Design review of the part built by this model. Coordinates are the model's own, in mm. Face numbers are marked on the shaded views. A direction names the side the tool comes from. Coordinates: 2 decimals unless noted, no trailing zeros. Order: outer loops, then holes, each group sorted by start corner. A loop starts at its lowest first (then second) coordinate and runs counter-clockwise, first axis right, second up. Notation, with made-up numbers: (30, -7) -> (65, -7) arc R21 cw to (65, 25) -> close; hole circle Ø2 at (71, -13). An arc over 180 degrees is marked (long way). Write item = value, one per line.
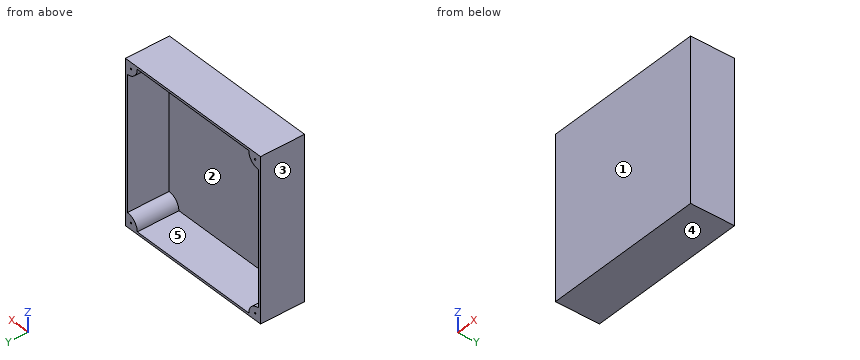
Autodesk Inventor part; units mm, degrees
ref_plane "YZ Plane" through (0, 0, 0) normal (1, 0, 0) x (0, 1, 0)
ref_plane "XZ Plane" through (0, 0, 0) normal (0, 1, 0) x (-1, 0, 0)
ref_plane "XY Plane" through (0, 0, 0) normal (0, 0, 1) x (1, 0, 0)
sketch "Boceto1" plane through (0, 0, 0) normal (0, 1, 0) x (-1, 0, 0)
  line L0 (-103, 103) -> (103, 103)
  line L1 (103, 103) -> (103, -103)
  line L2 (103, -103) -> (-103, -103)
  line L3 (-103, -103) -> (-103, 103)
  line L4 (-103, 103) -> (103, -103) construction
  line L5 (103, 103) -> (-103, -103) construction
  point P0 (0, 0)
  dimension "d0" = 206
  dimension "d1" = 206
extrude "Extrusión1" add sketch "Boceto1" along normal blind 56
shell "Vaciado1" thickness 3 removed faces 1 at (34.3333, 56, 34.3333)
sketch "Boceto2" plane through (-100, 3, -100) normal (0, 1, 0) x (1, 0, 0)
  line L0 (200, 0) -> (0, 0)
  arc A0 (0, -15) -> (15, 0) centre (0, 0) ccw
  line L1 (200, -200) -> (200, 0)
  arc A1 (185, 0) -> (200, -15) centre (200, 0) ccw
  line L2 (200, -200) -> (0, -200)
  arc A2 (200, -185) -> (185, -200) centre (200, -200) ccw
  line L3 (0, -200) -> (0, 0)
  arc A3 (15, -200) -> (0, -185) centre (0, -200) ccw
  line L4 (0, 0) -> (15, 0)
  line L5 (0, 0) -> (0, -15)
  line L6 (200, 0) -> (200, -15)
  line L7 (200, 0) -> (185, 0)
  line L8 (200, -200) -> (200, -185)
  line L9 (200, -200) -> (185, -200)
  line L10 (0, -200) -> (0, -185)
  line L11 (0, -200) -> (15, -200)
  point P0 (100, -100)
  dimension "d5" = 30
  dimension "d6" = 30
  dimension "d7" = 30
  dimension "d8" = 30
extrude "Extrusión2" add sketch "Boceto2" along normal blind 53 contours L1 A1 L0 | A0 L3 L0 | L1 L2 A2 | A3 L2 L3
sketch "Boceto3" plane through (0, 56, 0) normal (0, 1, 0) x (1, 0, 0)
  line L0 (85, 100) -> (103, 100)
  line L1 (103, -103) -> (103, 103)
  line L2 (100, -85) -> (100, 85)
  line L3 (100, 85) -> (100, 100)
  line L4 (100, 100) -> (116.202, 100) construction
  arc A0 (85, 100) -> (100, 85) centre (100, 100) ccw
  line L5 (89.3934, 89.3934) -> (89.3934, 100)
  line L6 (89.3934, 89.3934) -> (100, 89.3934)
  line L7 (89.3934, 100) -> (100, 89.3934)
  line L8 (89.3934, 89.3934) -> (100, 100)
  circle A1 centre (94.6967, 94.6967) radius 1
  circle A2 centre (-94.6967, 94.6967) radius 1
  circle A3 centre (-94.6967, -94.6967) radius 1
  circle A4 centre (94.6967, -94.6967) radius 1
  point P0 (0, 0)
  dimension "d12" = 2
  dimension "d15" = 360
hole "Agujero1" at (-94.6967, 56, -94.6967) at (-94.6967, 56, 94.6967) at (94.6967, 56, 94.6967) at (94.6967, 56, -94.6967) direction (0, -1, 0) diameter 2 depth 25 tip angle 118
properties part number "caja_cuboLed"
(1) The part is to be moulded in two halves that separate along X. For the marked faces 1, 2 and 3, say which applies: released by +X, released by -X, zero draft, split by the parting line, or undercut.
Report:
face_1 = zero draft
face_2 = undercut
face_3 = released by -X
(2) We need section C-C (z = 27.5). Write out the cut boundary in (x, y), and give its area (3 significant figures).
Report:
outline = (-103, 0) -> (103, 0) -> (103, 56) -> (100, 56) -> (100, 3) -> (-100, 3) -> (-100, 56) -> (-103, 56) -> close
area = 936 mm²
(3) Insertion check: pin 1 (1.6 mm diameter, centred on x = 94.7, z = 94.7, fed in from +Y). The pin has a flat end and moves straight along its axis. Give the tip position at first contact, or say it passes through.
Report:
pin_1 = 30.88
(4) For L1, parallel to X at y = 14, z = -35; L2, parallel to Y at x = 11.5, z = -87, list the stretches that pass through material, from the lowest coordinate up.
Report:
L1 = -103 to -100, 100 to 103
L2 = 0 to 3
(5) We need section B-B (x = 18). Write out the cut boundary in (y, z), and give its area (3 significant figures).
Report:
outline = (0, -103) -> (56, -103) -> (56, -100) -> (3, -100) -> (3, 100) -> (56, 100) -> (56, 103) -> (0, 103) -> close
area = 936 mm²
(6) For the marked faces 4 and 5, list the 3-axis set-ups (+Z, -Z, +X, -X, +Y, -Y) from which the entire face can be reached by the end or side of a thin tool; tool diameter is ignored.
Report:
face_4 = -Z, +X, -X, +Y, -Y
face_5 = +Y
(7) We need section A-A (y = 16). Write out the cut boundary in (x, z).
Report:
outline = (-103, -103) -> (103, -103) -> (103, 103) -> (-103, 103) -> close; hole (-100, -85) arc R15 cw to (-85, -100) -> (85, -100) arc R15 cw to (100, -85) -> (100, 85) arc R15 cw to (85, 100) -> (-85, 100) arc R15 cw to (-100, 85) -> close
(8) We need section D-D (y = 48.5). Write out the cut boundary in (x, z).
Report:
outline = (-103, -103) -> (103, -103) -> (103, 103) -> (-103, 103) -> close; hole (-100, -85) arc R15 cw to (-85, -100) -> (85, -100) arc R15 cw to (100, -85) -> (100, 85) arc R15 cw to (85, 100) -> (-85, 100) arc R15 cw to (-100, 85) -> close; hole circle Ø2 at (-94.7, -94.7); hole circle Ø2 at (-94.7, 94.7); hole circle Ø2 at (94.7, -94.7); hole circle Ø2 at (94.7, 94.7)
